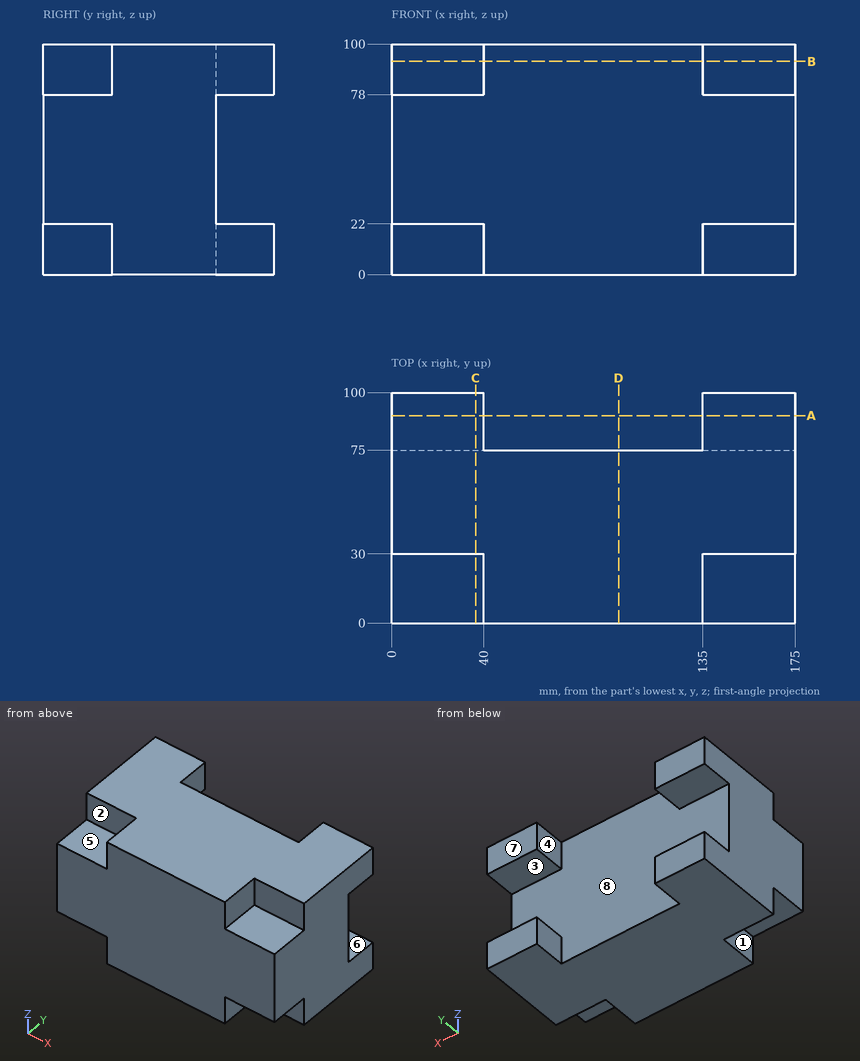
Print and shaded views of the part. All mm, measured from the part's lowest x, y and z. A direction names the side the tool comes from. Round coordinates to 2 decimals unless told otherwise and drop trailing zeros. Order: outer loops, then holes, each group sorted by start corner. A loop starts at its lowest first (then second) coordinate and runs counter-clockwise, first axis right, second up.
Q1. Slice it at C-C (x = 36.5). Write the cut outline in (y, z), and give its area (3 significant figures).
Q2. Slice it at B-B (z = 92.5). Write the cut outline in (x, y).
Q3. Drop flat-ended pins along their axis: pin 1 (1.5 mm diameter, centred on x = 80.5, z = 19, fed in from -Y); pin 2 (11 mm diameter, centred on x = 154.5, z = 94, fed in from -Y); pin 3 (11 mm diameter, centred on y = 16, z = 13.5, fed in from -X); pin 4 (6.5 mm diameter, centred on y = 13.5, z = 91, fed in from +X). Give the stop position or say it passes through.
Q4. Slice it at A-A (y = 90). Write the cut outline in (x, z).
Q5. Which spindle directions (+Z, -Z, +X, -X, +Y, -Y) get a long thin tool onto all of the face, cutting with end or side? Do the marked faces 1, 2, 3 and 4. Say none if no direction does.
Q6. Two-plate mould, pull along Z, no slides. Class the marked faces 5, 6, 7 and 8: pulls with the +Z half, pulls with the -Z half, needs draft (parallel to the pull), parting line crosses it, or undercut.
Q7. Slice it at D-D (x = 98.5). Write the cut outline in (y, z).
Q8. Wall check: L1, parallel to X at y = 77.5, z = 13; L2, parallel to Z at x = 35, y = 95.5; L3, parallel to Y at x = 157, z = 43.5. Give the ranges that are in metal, low to high.
Results below:
1. outline: (0, 22) - (30, 22) - (30, 0) - (100, 0) - (100, 22) - (75, 22) - (75, 78) - (100, 78) - (100, 100) - (30, 100) - (30, 78) - (0, 78) - close
1. area: 7,280 mm2
2. outline: (0, 30) - (40, 30) - (40, 0) - (135, 0) - (135, 30) - (175, 30) - (175, 100) - (135, 100) - (135, 75) - (40, 75) - (40, 100) - (0, 100) - close
3. pin 1: stops at y = 0
3. pin 2: stops at y = 30
3. pin 3: stops at x = 40
3. pin 4: stops at x = 135
4. outline: (0, 0) - (40, 0) - (40, 22) - (0, 22) - close; (0, 78) - (40, 78) - (40, 100) - (0, 100) - close; (135, 0) - (175, 0) - (175, 22) - (135, 22) - close; (135, 78) - (175, 78) - (175, 100) - (135, 100) - close
5. face 1: -Z, -X, -Y
5. face 2: +Z, -X, -Y
5. face 3: +X, -X, +Y
5. face 4: +Z, -Z, +Y
6. face 5: pulls with the +Z half
6. face 6: undercut
6. face 7: needs draft
6. face 8: undercut
7. outline: (0, 0) - (75, 0) - (75, 100) - (0, 100) - close
8. L1: x = 0 to 40, 135 to 175
8. L2: z = 0 to 22, 78 to 100
8. L3: y = 0 to 75
